CAD build for the part. Positions are in the model's coordinates, mm. Round coordinates to 2 decimals unless told otherwise and drop trailing zeros. Order: outer loops, then holes, each group sorted by start corner. A loop starts at its lowest first (then second) coordinate and runs counter-clockwise, first axis right, second up. Notation, with made-up numbers: M -25,40.25 L 34,40.25 A31 cw 34,66.25 Z; hole C 73,78 d6. An arc over 180 degrees is marked long. Answer as a JSON object with one key per item and string values.
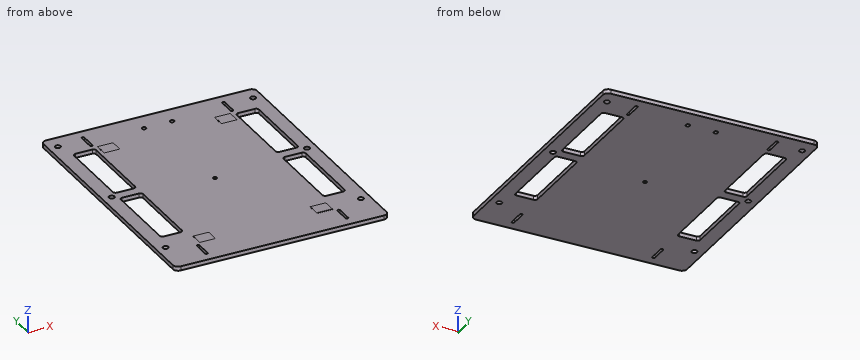
```python
from build123d import *

# Parameters (mm, degrees)
BOSS_EXTRUDE1_DEPTH = 1.6
SKETCH2_R           = 0.75
SKETCH2_R_2         = 1.05
SKETCH2_R_3         = 0.8
CUT_EXTRUDE1_DEPTH  = 65.680445267
CUT_EXTRUDE2_DEPTH  = 65.680445267
CUT_EXTRUDE3_DEPTH  = 1.6
SKETCH5_W           = 6
SKETCH5_H           = 5
BOSS_EXTRUDE2_DEPTH = 0.02


with BuildPart() as part:
    # Sketch1 → Boss-Extrude1 (new body)
    with BuildSketch(Plane.XY):
        with BuildLine():
            Line((-39, -50), (39, -50))
            ThreePointArc((39, -50), (40.414213562, -49.414213562), (41, -48))
            Line((41, -48), (41, 48))
            ThreePointArc((41, 48), (40.414213562, 49.414213562), (39, 50))
            Line((39, 50), (-39, 50))
            ThreePointArc((-39, 50), (-40.414213562, 49.414213562), (-41, 48))
            Line((-41, 48), (-41, -48))
            ThreePointArc((-41, -48), (-40.414213562, -49.414213562), (-39, -50))
        make_face()
    extrude(amount=BOSS_EXTRUDE1_DEPTH)

    # Sketch2 → Cut-Extrude1 (cut, through all)
    with BuildSketch(Plane.XY.offset(1.6)):
        Circle(SKETCH2_R)
        with Locations((-37.5, 44.2)):
            Circle(SKETCH2_R_2)
        with Locations((37.5, 44.2)):
            Circle(SKETCH2_R_2)
        with Locations((37.5, 4.2)):
            Circle(SKETCH2_R_2)
        with Locations((37.5, -35.8)):
            Circle(SKETCH2_R_2)
        with Locations((-37.5, 4.2)):
            Circle(SKETCH2_R_2)
        with Locations((-37.5, -35.8)):
            Circle(SKETCH2_R_2)
        with Locations((-5.38, 42.25)):
            Circle(SKETCH2_R_3)
        with Locations((5.39, 42.25)):
            Circle(SKETCH2_R_3)
    extrude(amount=-CUT_EXTRUDE1_DEPTH, mode=Mode.SUBTRACT)

    # Sketch3 → Cut-Extrude2 (cut, through all)
    with BuildSketch(Plane.XY.offset(1.6)):
        with BuildLine():
            Line((-34.5, 37), (-28, 37))
            ThreePointArc((-28, 37), (-27.292893219, 36.707106781), (-27, 36))
            Line((-27, 36), (-27, 7.2))
            ThreePointArc((-27, 7.2), (-27.292893219, 6.492893219), (-28, 6.2))
            Line((-28, 6.2), (-34.5, 6.2))
            ThreePointArc((-34.5, 6.2), (-35.207106781, 6.492893219), (-35.5, 7.2))
            Line((-35.5, 7.2), (-35.5, 36))
            ThreePointArc((-35.5, 36), (-35.207106781, 36.707106781), (-34.5, 37))
        make_face()
        with BuildLine():
            Line((28, 37), (34.5, 37))
            ThreePointArc((34.5, 37), (35.207106781, 36.707106781), (35.5, 36))
            Line((35.5, 36), (35.5, 7.2))
            ThreePointArc((35.5, 7.2), (35.207106781, 6.492893219), (34.5, 6.2))
            Line((34.5, 6.2), (28, 6.2))
            ThreePointArc((28, 6.2), (27.292893219, 6.492893219), (27, 7.2))
            Line((27, 7.2), (27, 36))
            ThreePointArc((27, 36), (27.292893219, 36.707106781), (28, 37))
        make_face()
        with BuildLine():
            Line((28, 2.2), (34.5, 2.2))
            ThreePointArc((34.5, 2.2), (35.207106781, 1.907106781), (35.5, 1.2))
            Line((35.5, 1.2), (35.5, -27.6))
            ThreePointArc((35.5, -27.6), (35.207106781, -28.307106781), (34.5, -28.6))
            Line((34.5, -28.6), (28, -28.6))
            ThreePointArc((28, -28.6), (27.292893219, -28.307106781), (27, -27.6))
            Line((27, -27.6), (27, 1.2))
            ThreePointArc((27, 1.2), (27.292893219, 1.907106781), (28, 2.2))
        make_face()
        with BuildLine():
            Line((-34.5, 2.2), (-28, 2.2))
            ThreePointArc((-28, 2.2), (-27.292893219, 1.907106781), (-27, 1.2))
            Line((-27, 1.2), (-27, -27.6))
            ThreePointArc((-27, -27.6), (-27.292893219, -28.307106781), (-28, -28.6))
            Line((-28, -28.6), (-34.5, -28.6))
            ThreePointArc((-34.5, -28.6), (-35.207106781, -28.307106781), (-35.5, -27.6))
            Line((-35.5, -27.6), (-35.5, 1.2))
            ThreePointArc((-35.5, 1.2), (-35.207106781, 1.907106781), (-34.5, 2.2))
        make_face()
    extrude(amount=-CUT_EXTRUDE2_DEPTH, mode=Mode.SUBTRACT)

    # Sketch4 → Cut-Extrude3 (cut)
    with BuildSketch(Plane.XY.offset(1.6)):
        with BuildLine():
            Line((-27.5, 39.75), (-27.5, 45.75))
            ThreePointArc((-27.5, 45.75), (-27, 46.25), (-26.5, 45.75))
            Line((-26.5, 45.75), (-26.5, 39.75))
            ThreePointArc((-26.5, 39.75), (-27, 39.25), (-27.5, 39.75))
        make_face()
        with BuildLine():
            Line((26.5, 39.75), (26.5, 45.75))
            ThreePointArc((26.5, 45.75), (27, 46.25), (27.5, 45.75))
            Line((27.5, 45.75), (27.5, 39.75))
            ThreePointArc((27.5, 39.75), (27, 39.25), (26.5, 39.75))
        make_face()
        with BuildLine():
            Line((26.5, -45.75), (26.5, -39.75))
            ThreePointArc((26.5, -39.75), (27, -39.25), (27.5, -39.75))
            Line((27.5, -39.75), (27.5, -45.75))
            ThreePointArc((27.5, -45.75), (27, -46.25), (26.5, -45.75))
        make_face()
        with BuildLine():
            Line((-27.5, -45.75), (-27.5, -39.75))
            ThreePointArc((-27.5, -39.75), (-27, -39.25), (-26.5, -39.75))
            Line((-26.5, -39.75), (-26.5, -45.75))
            ThreePointArc((-26.5, -45.75), (-27, -46.25), (-27.5, -45.75))
        make_face()
    extrude(amount=-CUT_EXTRUDE3_DEPTH, mode=Mode.SUBTRACT)

    # Sketch5 → Boss-Extrude2 (add)
    with BuildSketch(Plane.XY.offset(1.6)):
        with Locations((-22.5, 35.5)):
            Rectangle(SKETCH5_W, SKETCH5_H)
        with Locations((22.5, 35.5)):
            Rectangle(SKETCH5_W, SKETCH5_H)
        with Locations((22.5, -35.5)):
            Rectangle(SKETCH5_W, SKETCH5_H)
        with Locations((-22.5, -35.5)):
            Rectangle(SKETCH5_W, SKETCH5_H)
    extrude(amount=BOSS_EXTRUDE2_DEPTH)


solid = part.part
```
Item 1: Drop a flat-ended pin along its axis: pin 1 Ø5 at (x, y) = (-2, 30.5) entering from +Z. Give the stop position or say it passes through.
Worked answers:
{"pin 1": "stops at z = 1.6"}
Item 2: Saw through at A-A on y = 4.2. List the corners of the cut face in (x, z).
Worked answers:
{"outline": "M -41,0 L -38.55,0 L -38.55,1.6 L -41,1.6 Z; M -36.45,0 L 36.45,0 L 36.45,1.6 L -36.45,1.6 Z; M 38.55,0 L 41,0 L 41,1.6 L 38.55,1.6 Z"}
Item 3: Saw through at C-C on z = 0.35. State how many separate pieces and enclosed holes the cut face has, and give its area (3 significant figures).
Worked answers:
{"separate pieces": "1", "enclosed holes": "17", "area": "7,100 mm2"}
Item 4: Saw through at B-B on x = 30. List the corners of the cut face in (y, z).
Worked answers:
{"outline": "M -50,0 L -28.6,0 L -28.6,1.6 L -50,1.6 Z; M 2.2,0 L 6.2,0 L 6.2,1.6 L 2.2,1.6 Z; M 37,0 L 50,0 L 50,1.6 L 37,1.6 Z"}
Item 5: Wall check: line 1 along X through (y, z) = (42.25, 0.5); line 2 along X through (y, z) = (28.5, 0.4); line 3 along Y through (x, z) = (37.5, 0.5). Give the ranges that are in metal, low to high. Write a range as [from, to].
Worked answers:
{"line 1": "x = [-41, -27.5], [-26.5, -6.18], [-4.58, 4.59], [6.19, 26.5], [27.5, 41]", "line 2": "x = [-41, -35.5], [-27, 27], [35.5, 41]", "line 3": "y = [-50, -36.85], [-34.75, 3.15], [5.25, 43.15], [45.25, 50]"}
